Geometry: final body of the model. Coordinates: model frame, mm. A direction names the side the tool comes from. Coordinates: 2 decimals unless noted, no trailing zeros. Loops run counter-clockwise (first coordinate to the right, second up) from the corner with the lowest first, then second, coordinate; pieces in that order, holes last. Notation, with made-up numbers: M -29,49 L 7,49 A27 ccw 7,83 Z; hole C -11.5,1.25 d9. An arc over 180 degrees is marked long. Write each question's results on one line, items separated by ' | '. Start each with the question number.
from build123d import *

# Parameters (mm, degrees)
SKETCH1_R           = 125
BOSS_EXTRUDE1_DEPTH = 900
SKETCH2_R           = 10
CUT_EXTRUDE1_DEPTH  = 350
SKETCH3_R           = 10
CUT_EXTRUDE2_DEPTH  = 400


with BuildPart() as part:
    # Sketch1 → Boss-Extrude1 (new body)
    with BuildSketch(Plane.XY):
        Circle(SKETCH1_R)
    extrude(amount=BOSS_EXTRUDE1_DEPTH)

    # Sketch2 → Cut-Extrude1 (cut)
    with BuildSketch(Plane.XY.offset(900)):
        Circle(SKETCH2_R)
    extrude(amount=-CUT_EXTRUDE1_DEPTH, mode=Mode.SUBTRACT)

    # Sketch3 → Cut-Extrude2 (cut)
    with BuildSketch(Plane(origin=(0, 0, 0), x_dir=(-1, 0, 0), z_dir=(0, 0, -1))):
        Circle(SKETCH3_R)
    extrude(amount=-CUT_EXTRUDE2_DEPTH, mode=Mode.SUBTRACT)


solid = part.part
Item 1: Section A-A, the plane x = 0. Return loops of the section in (y, z).
Item 2: Section D-D, the plane x = 65. Return loops of the section in (y, z), plus the area to 3 significant figures.
Item 3: Ray query, L1, parallel to Y at x = 0, z = 667; L2, parallel to X at y = 2, z = 537; L3, parallel to X at y = -3, z = 300. Return the intervals inside material, ascending. Write a range as [from, to].
Item 4: Section C-C, the plane z = 224. Return loops of the section in (x, y), plus the area to 3 significant figures.
Item 5: Set-up query: faces 1 (the flat face through (0, 0, 550)), 2 (the cylindrical face through (2.17, -9.76, 197.2)), 3 (the flat face through (-2, -26, 900)). Return all of +Z, -Z, +X, -X, +Y, -Y with unobstructed straight access to the full face (end or side cutting, diameter ignored); none if empty.
Item 6: Contact query for flat-ended pins moving along their axis: P1, Ø16, axis at x = -0.5, y = 2, coming from the -Z side; P2, Ø1.5, axis at y = -85.5, z = 126, coming from the +X side; P3, Ø6, axis at x = 3, y = -5, coming from the +Z side; P4, Ø12, axis at x = 50, z = 379, coming from the +Y side. Output: stop coordinate, or through.
Item 7: Pull-direction query (Y, two-part tool) for faces 4 (the cylindrical face through (-2.17, -9.76, 727.45)), 5 (the cylindrical face through (-124.88, 5.5, 443.7)), 6 (the flat face through (-2, -26, 0)); classes: released by +Y, released by -Y, zero draft, split by the parting line, or undercut.
Solutions:
1) outline: M -125,0 L -10,0 L -10,400 L 10,400 L 10,0 L 125,0 L 125,900 L 10,900 L 10,550 L -10,550 L -10,900 L -125,900 Z
2) outline: M -106.77,0 L 106.77,0 L 106.77,900 L -106.77,900 Z | area: 192,000 mm²
3) L1: y = [-125, -10], [10, 125] | L2: x = [-124.98, 124.98] | L3: x = [-124.96, -9.54], [9.54, 124.96]
4) outline: C 0,0 d250; hole C 0,0 d20 | area: 48,800 mm²
5) face 1: +Z | face 2: -Z | face 3: +Z, +X, -X, +Y, -Y
6) P1: stops at z = 0 | P2: stops at x = 91.88 | P3: stops at z = 550 | P4: stops at y = 117
7) face 4: undercut | face 5: split by the parting line | face 6: zero draft
